The model under review builds one solid part; all positions refer to its coordinate system, in mm. A direction names the side the tool comes from. Round coordinates to 2 decimals unless told otherwise and drop trailing zeros. Write each loop counter-clockwise with the first axis right and the second up, starting at its lowest first coordinate (ties: lowest second). Pieces come first, ordered by that corner, then holes. Notation, with made-up numbers: (26, 30.5) -> (48, 30.5) arc R29 cw to (48, 60.5) -> close; hole circle Ø5 at (12.5, 19). An arc over 180 degrees is marked (long way). Return JSON: item names as keys, results as strings. Group by question number.
1. For line 1 along Y through (x, z) = (49.25, 0); line 2 along Z through (x, y) = (6, -0.25); line 3 along Z through (x, y) = (-32, 3.5), list the stretches that pass through material, from the lowest coordinate up. Write a range as from..to.
2. Take a section at B-B, the plane y = -3. Write out the cut boundary in (x, z).
3. Take a section at C-C, the plane z = 2.5. Write out the cut boundary in (x, y), then the cut area to 3 significant figures.
4. Clearance check with flat-ended pins moving along their axes: P1, Ø1, axis at x = -9.5, y = -3, coming from the -Z side; P2, Ø2, axis at y = 0, z = 0, coming from the +X side; P3, Ø4, axis at x = 32, z = 2.5, coming from the +Y side. State where each tip first meets the part, or that it passes through.
5. Take a section at A-A, the plane x = 2. Write out the cut boundary in (y, z), then the cut area to 3 significant figures.
6. Tool access review of faces 1 (the flat face through (-61.25, 1, -1)), 2 (the cylindrical face through (-50.65, 1.22, 0.27)): name each direction out of +Z, -Z, +X, -X, +Y, -Y from which nothing blocks a thin tool from reaching the whole face with its end or side.
7. Mouldability with a two-part tool opening along Y and no side actions: class faces 3 (the cylindrical face through (0.858, -3.905, 0.867)), 4 (the flat face through (61.25, 1, -1)), 5 (the cylindrical face through (50.65, 1.22, 0.27)) as pulls with the +Y half, pulls with the -Y half, needs draft (parallel to the pull), parting line crosses it, or undercut.
from build123d import *

# Parameters (mm, degrees)
SKETCH_2_R      = 4
EXTRUDE_1_DEPTH = 61.25


with BuildPart() as part:
    # 스케치2 → 보스-돌출1 (new body)
    with BuildSketch(Plane(origin=(0, 0, 0), x_dir=(0, 0, -1), z_dir=(1, 0, 0))):
        Circle(SKETCH_2_R)
    extrude_1 = extrude(amount=EXTRUDE_1_DEPTH)

    # 스케치4 → M3x0.5 나사 구멍1 (revolve, cut)
    with BuildSketch(Plane(origin=(61.25, 0, 0), x_dir=(0, 0, -1), z_dir=(0, 1, 0))):
        Polygon((0, 0), (0, 22.251075774), (1.25, 21.5), (1.25, 0), align=None)
    m3x0_5_1 = revolve(axis=Axis((67.6, 0, 0), (-1, 0, 0)), mode=Mode.SUBTRACT)

    # 대칭 복사1: 보스-돌출1, M3x0.5 나사 구멍1 across plane
    add(extrude_1.mirror(Plane(origin=(0, 0, 0), x_dir=(0, 0, 1), z_dir=(1, 0, 0))))
    add(m3x0_5_1.mirror(Plane(origin=(0, 0, 0), x_dir=(0, 0, 1), z_dir=(1, 0, 0))), mode=Mode.SUBTRACT)


solid = part.part
Output:
{
 "1": {"line 1": "y = -4..-1.25, 1.25..4", "line 2": "z = -3.99..3.99", "line 3": "z = -1.94..1.94"},
 "2": {"outline": "(-61.25, -2.65) -> (61.25, -2.65) -> (61.25, 2.65) -> (-61.25, 2.65) -> close"},
 "3": {"outline": "(-61.25, -3.12) -> (61.25, -3.12) -> (61.25, 3.12) -> (-61.25, 3.12) -> close", "area": "765 mm^2"},
 "4": {"P1": "stops at z = -3.12", "P2": "stops at x = 39.6", "P3": "stops at y = 3.97"},
 "5": {"outline": "circle Ø8 at (0, 0)", "area": "50.3 mm^2"},
 "6": {"face 1": "+Z, -Z, -X, +Y, -Y", "face 2": "-X"},
 "7": {"face 3": "parting line crosses it", "face 4": "needs draft", "face 5": "undercut"}
}
